from build123d import *

# Parameters (mm, degrees)
SKETCH1_W                                            = 16.1
SKETCH1_H                                            = 14.1
BOSS_EXTRUDE1_DEPTH                                  = 7
SKETCH3_W                                            = 12.1
SKETCH3_H                                            = 10.1
CUT_EXTRUDE1_DEPTH                                   = 5
CSK_FOR_M1_6_COUNTERSUNK_FLAT_HEAD_SCREW_D           = 2
CSK_FOR_M1_6_COUNTERSUNK_FLAT_HEAD_SCREW_DEPTH       = 2
CSK_FOR_M1_6_COUNTERSUNK_FLAT_HEAD_SCREW_CSINK_D     = 4
CSK_FOR_M1_6_COUNTERSUNK_FLAT_HEAD_SCREW_CSINK_ANGLE = 90
SKETCH8_R                                            = 2.25
CUT_EXTRUDE2_DEPTH                                   = 3
FILLET1_R                                            = 2
FILLET2_R                                            = 0.2


with BuildPart() as part:
    # Sketch1 → Boss-Extrude1 (new body)
    with BuildSketch(Plane(origin=(0, 0, 0), x_dir=(1, 0, 0), z_dir=(0, 1, 0))):
        Rectangle(SKETCH1_W, SKETCH1_H)
    extrude(amount=BOSS_EXTRUDE1_DEPTH)

    # Sketch3 → Cut-Extrude1 (cut)
    with BuildSketch(Plane(origin=(0, 7, 0), x_dir=(1, 0, 0), z_dir=(0, 1, 0))):
        Rectangle(SKETCH3_W, SKETCH3_H)
    extrude(amount=-CUT_EXTRUDE1_DEPTH, mode=Mode.SUBTRACT)

    # CSK for M1.6 Countersunk Flat Head Screw1
    with Locations(Plane(origin=(0, 0, 0), x_dir=(-1, 0, 0), z_dir=(0, -1, 0))):
        with Locations((4.5, 0), (-4.5, 0)):
            CounterSinkHole(CSK_FOR_M1_6_COUNTERSUNK_FLAT_HEAD_SCREW_D / 2, CSK_FOR_M1_6_COUNTERSUNK_FLAT_HEAD_SCREW_CSINK_D / 2, depth=CSK_FOR_M1_6_COUNTERSUNK_FLAT_HEAD_SCREW_DEPTH, counter_sink_angle=CSK_FOR_M1_6_COUNTERSUNK_FLAT_HEAD_SCREW_CSINK_ANGLE)

    # Sketch8 → Cut-Extrude2 (cut, through all)
    with BuildSketch(Plane(origin=(0, 2, 0), x_dir=(1, 0, 0), z_dir=(0, 1, 0))):
        Circle(SKETCH8_R)
    extrude(amount=-CUT_EXTRUDE2_DEPTH, mode=Mode.SUBTRACT)

    # Fillet1
    fillet1_edges = [part.edges().sort_by_distance(p)[0] for p in [
        (-8.05, 3.5, -7.05),
        (8.05, 3.5, -7.05),
        (8.05, 3.5, 7.05),
        (-8.05, 3.5, 7.05),
    ]]
    fillet(fillet1_edges, radius=FILLET1_R)

    # Fillet2
    fillet2_edges = [part.edges().sort_by_distance(p)[0] for p in [
        (-6.05, 4.5, 5.05),
        (-6.05, 4.5, -5.05),
        (6.05, 4.5, -5.05),
        (6.05, 4.5, 5.05),
    ]]
    fillet(fillet2_edges, radius=FILLET2_R)


solid = part.part
The listing builds one solid part. Answer for the finished solid, in the listing's coordinates (mm). A direction names the side the tool comes from. Give positions to 0.01 mm unless a question says otherwise; leave off trailing zeros. Write each loop counter-clockwise with the first axis right and the second up, starting at its lowest first coordinate (ties: lowest second). Pieces come first, ordered by that corner, then holes. Notation, with made-up numbers: (7, 61) - (21, 61) arc R16 cw to (21, 86) - close; hole circle Ø1 at (81, 13.5). An arc over 180 degrees is marked (long way). One line per question, with ' | ' between items. Start each with the question number.
1. Section C-C, the plane z = 0 is taken. Determine the outline of the cut face in (x, y).
2. Straight lines are drawn through the part: line 1 (Z direction, x = 4.5, y = 1.75); line 2 (Z direction, x = 0.75, y = 6); line 3 (X direction, y = 6, z = 2). For each, find the intervals that lie inside material, in ascending order.
3. Given P1, Ø3, axis at x = 2.5, z = -0.5, coming from the +Y side, flat-ended and moving along its own axis, determine where the tip first touches the part or whether it passes through.
4. Determine the mould class of faces 1 (the face through (0, 7, 6)), 2 (the face through (0, 3, -7.05)), 3 (the face through (-1.4, 2, -2.3)) for opening direction Z: +Z half, -Z half, draft (parallel to the pull), parting line (faces both ways), or undercut.
5. For faces 4 (the face through (6.05, 5, 0)), 5 (the face through (7.45, 3.55, 6.48)), determine the directions among +Z, -Z, +X, -X, +Y, -Y from which every point of the face is accessible in a straight line to the end or side of a thin tool.
6. Section B-B, the plane y = 3.25 is taken. Determine the outline of the cut face in (x, z).
7. Section D-D, the plane z = 4 is taken. Determine the outline of the cut face in (x, y), then the cut area to 3 significant figures.
8. Section A-A, the plane x = 0 is taken. Determine the outline of the cut face in (y, z), then the cut area to 3 significant figures.
Result:
1) outline: (-8.05, 0) - (-6.5, 0) - (-5.5, 1) - (-5.5, 2) - (-6.05, 2) - (-6.05, 7) - (-8.05, 7) - close; (-3.5, 1) - (-2.5, 0) - (-2.25, 0) - (-2.25, 2) - (-3.5, 2) - close; (2.25, 0) - (2.5, 0) - (3.5, 1) - (3.5, 2) - (2.25, 2) - close; (5.5, 1) - (6.5, 0) - (8.05, 0) - (8.05, 7) - (6.05, 7) - (6.05, 2) - (5.5, 2) - close
2) line 1: z = -7.05 to -1, 1 to 7.05 | line 2: z = -7.05 to -5.05, 5.05 to 7.05 | line 3: x = -8.05 to -6.05, 6.05 to 8.05
3) P1: stops at y = 2
4) face 1: draft | face 2: -Z half | face 3: undercut
5) face 4: +Y | face 5: +Z, +X, +Y, -Y
6) outline: (-8.05, -5.05) arc R2 ccw to (-6.05, -7.05) - (6.05, -7.05) arc R2 ccw to (8.05, -5.05) - (8.05, 5.05) arc R2 ccw to (6.05, 7.05) - (-6.05, 7.05) arc R2 ccw to (-8.05, 5.05) - close; hole (-6.05, -4.85) arc R0.2 ccw to (-5.85, -5.05) - (5.85, -5.05) arc R0.2 ccw to (6.05, -4.85) - (6.05, 4.85) arc R0.2 ccw to (5.85, 5.05) - (-5.85, 5.05) arc R0.2 ccw to (-6.05, 4.85) - close
7) outline: (-8.05, 0) - (8.05, 0) - (8.05, 7) - (6.05, 7) - (6.05, 2) - (-6.05, 2) - (-6.05, 7) - (-8.05, 7) - close | area: 52.2 mm2
8) outline: (0, -7.05) - (7, -7.05) - (7, -5.05) - (2, -5.05) - (2, -2.25) - (0, -2.25) - close; (0, 2.25) - (2, 2.25) - (2, 5.05) - (7, 5.05) - (7, 7.05) - (0, 7.05) - close | area: 39.2 mm2
